Geometry: see drawing. Coordinates: mm, zero at the bounding-box minimum. Give positions to 0.01 mm unless a question says otherwise; leave off trailing zeros. Order: outer loops, then holes, each group sorted by start corner. A loop starts at its lowest first (then second) coordinate and runs counter-clockwise, first axis right, second up. Notation, with made-up numbers: (4.5, 65.5) - (33.5, 65.5) arc R34 ccw to (33.5, 100.5) - close; hole circle Ø10 at (23.5, -20). An arc over 180 degrees is marked (long way). Put each result on its own line as item: value. Start each with the question number.
1. Section D-D on x = 15.5. Return the cut outline in (y, z).
2. Ray query, line 1 along X through (y, z) = (40.5, 2.65); line 2 along X through (y, z) = (82.5, 1.2); line 3 along Y through (x, z) = (44, 0.2). Return the intervals inside material, ascending. Write a range as from..to.
3. Section A-A on x = 55. Return the cut outline in (y, z).
4. First-contact query: P1, Ø2, axis at x = 63.5, z = 0.5, coming from the -Y side; P2, Ø1.2, axis at y = 47, z = 1, coming from the -X side; P3, Ø1.5, axis at x = 99.5, z = 3.5, coming from the -Y side; P4, Ø10, axis at x = 43.5, y = 32.5, coming from the +Z side. Flat tips, straight axial feed; report the tip coordinate or a pass-through.
5. Section B-B on y = 68.5. Return the cut outline in (x, z).
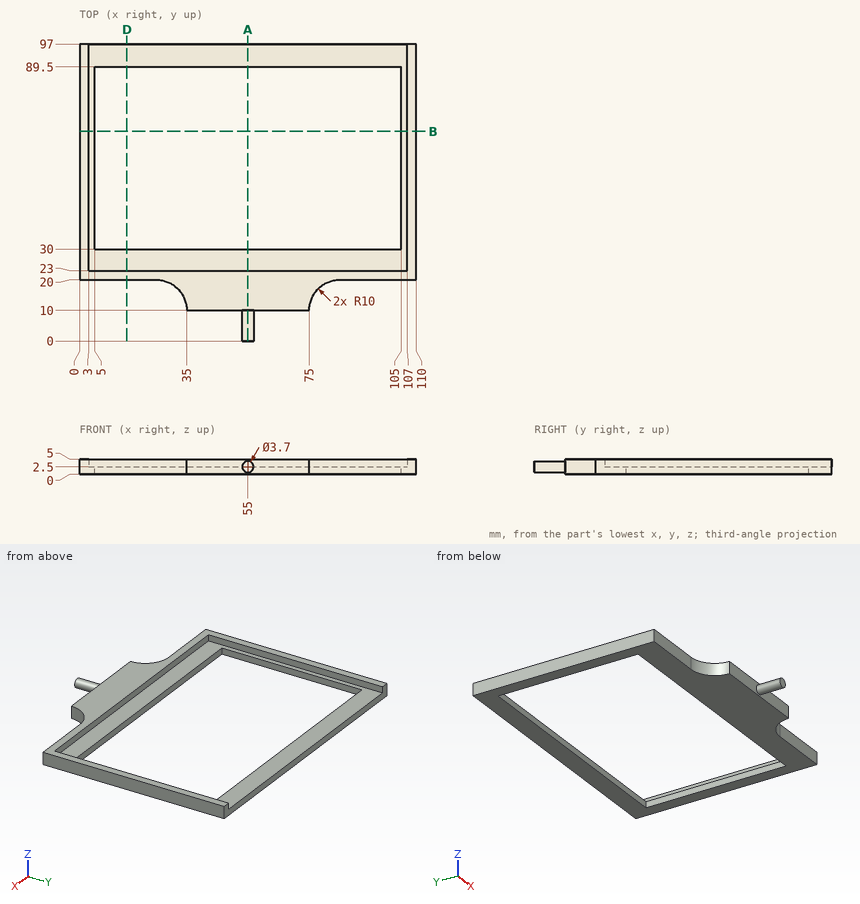
Resolved:
1. outline: (20, 0) - (30, 0) - (30, 2.5) - (23, 2.5) - (23, 5) - (20, 5) - close; (89.5, 0) - (97, 0) - (97, 2.5) - (89.5, 2.5) - close
2. line 1: 0..3, 107..110
2. line 2: 0..5, 105..110
2. line 3: 10..30, 89.5..97
3. outline: (0, 0.65) - (10, 0.65) - (10, 0) - (30, 0) - (30, 2.5) - (23, 2.5) - (23, 5) - (10, 5) - (10, 4.35) - (0, 4.35) - close; (89.5, 0) - (97, 0) - (97, 2.5) - (89.5, 2.5) - close
4. P1: y = 10
4. P2: x = 0
4. P3: y = 20
4. P4: z = 2.5
5. outline: (0, 0) - (5, 0) - (5, 2.5) - (3, 2.5) - (3, 5) - (0, 5) - close; (105, 0) - (110, 0) - (110, 5) - (107, 5) - (107, 2.5) - (105, 2.5) - close
